```python
from build123d import *

# Parameters (mm, degrees)
F0_W     = 107.6
F0_H     = 53
F1_DEPTH = 14.5
F2_W     = 105.6
F2_H     = 52
F3_DEPTH = 14
F4_SIZE  = 9
F5_W     = 11
F5_H     = 3.2
F6_DEPTH = 1
F7_W     = 15
F7_H     = 6
F8_DEPTH = 1
F9_R     = 2
F10_R    = 4


with BuildPart() as f1:
    # F0 (on Top) → F1 (new body)
    with BuildSketch(Plane.XY):
        Rectangle(F0_W, F0_H)
    extrude(amount=F1_DEPTH)

    # F2 (on face) → F3 (cut)
    with BuildSketch(Plane.XY.offset(14.5)):
        with Locations((0, -0.5)):
            Rectangle(F2_W, F2_H)
    extrude(amount=-F3_DEPTH, mode=Mode.SUBTRACT)

    # F4
    f4_edges = [f1.edges().sort_by_distance(p)[0] for p in [
        (53.8, 0, 0),
        (0, 26.5, 0),
        (-53.8, 0, 0),
        (-52.8, -0.5, 0.5),
        (0, 25.5, 0.5),
        (52.8, -0.5, 0.5),
    ]]
    chamfer(f4_edges, length=F4_SIZE)

    # F5 (on face) → F6 (join)
    with BuildSketch(Plane.XY.offset(14.5)):
        with Locations((-25, 27.1)):
            Rectangle(F5_W, F5_H)
        with Locations((25, 27.1)):
            Rectangle(F5_W, F5_H)
    extrude(amount=F6_DEPTH)

    # F7 (on face) → F8 (join)
    with BuildSketch(Plane.XY.offset(0.5)):
        with Locations((-21.7, -26.5)):
            Rectangle(F7_W, F7_H)
        with Locations((21.7, -26.5)):
            Rectangle(F7_W, F7_H)
    extrude(amount=F8_DEPTH)

    # F9
    f9_edges = [f1.edges().sort_by_distance(p)[0] for p in [
        (-29.2, -29.5, 1),
        (-14.2, -29.5, 1),
        (14.2, -29.5, 1),
        (29.2, -29.5, 1),
        (29.2, -23.5, 1),
        (14.2, -23.5, 1),
        (-29.2, -23.5, 1),
        (-14.2, -23.5, 1),
        (30.5, 28.7, 15),
        (19.5, 28.7, 15),
        (-19.5, 28.7, 15),
        (-30.5, 28.7, 15),
    ]]
    fillet(f9_edges, radius=F9_R)

    # F10
    f10_edges = [f1.edges().sort_by_distance(p)[0] for p in [
        (53.8, 26.5, 11.75),
        (52.8, 25.5, 12),
        (-52.8, 25.5, 12),
        (-53.8, 26.5, 11.75),
    ]]
    fillet(f10_edges, radius=F10_R)


solid = f1.part
```
Geometry check sheet. Reference: the model listing, model coordinates, mm. A direction names the side the tool comes from. Coordinates: 2 decimals unless noted, no trailing zeros. Order: outer loops, then holes, each group sorted by start corner. A loop starts at its lowest first (then second) coordinate and runs counter-clockwise, first axis right, second up. Notation, with made-up numbers: (45, 42) - (99, 42) arc R16 cw to (99, 49) - close; hole circle Ø4 at (70.25, 72). An arc over 180 degrees is marked (long way). Answer in a Markdown table with one row per item. Add a question column.
1. Section check C-C (z = 4.5). Enter the section's corners in (x, y), plus the area to 3 significant figures.
2. Draft check along X on faces 1 (the face through (14.8, -24.07, 1.01)), 2 (the face through (-1, -5, 0.5)), 3 (the face through (52.659, 25.297, 11.211)), 4 (the face through (-53.8, -2, 12)). Enter one of: +X half, -X half, draft (parallel to the pull), parting line (faces both ways), or undercut.
3. Section check D-D (x = 32.5). Enter the section's corners in (y, z).
4. Material ranges on L1, parallel to X at y = 6, z = 10.75; L2, parallel to Y at x = -48.5, z = 12.5; L3, parallel to Z at x = 15, y = -20, recorded low to high. Write a range as [from, to].
5. Gauge pin test, flat ends, axial feed: pin 1 Ø1 at (y, z) = (7.5, 3) entering from +X; pin 2 Ø0.5 at (y, z) = (-26.5, 1) entering from -X; pin 3 Ø0.5 at (y, z) = (-26.5, 1) entering from +X. Record the tip position at first contact, or that the pin passes through.
6. Access from +Z, -Z, +X, -X, +Y, -Y to the whole of each face (thin tool, end or side, straight path). Record for faces 5 (the face through (-48.4, -1.4, 5.1)), 6 (the face through (-14.8, -24.07, 1.01)), 7 (the face through (20.07, 28.1, 15.01)), 8 (the face through (25, 28, 14.5)).
7. Section check A-A (y = -6). Enter the section's corners in (x, z).
8. Section check B-B (x = -17.5). Enter the section's corners in (y, z), plus the area to 3 significant figures.
Data:
| question | item | result |
|---|---|---|
| 1 | outline | (-49.3, -26.5) - (-47.8, -26.5) - (-47.8, 20.5) - (47.8, 20.5) - (47.8, -26.5) - (49.3, -26.5) - (49.3, 22) - (-49.3, 22) - close |
| 1 | area | 289 mm² |
| 2 | face 1 | undercut |
| 2 | face 2 | undercut |
| 2 | face 3 | +X half |
| 2 | face 4 | -X half |
| 3 | outline | (-26.5, 0) - (17.5, 0) - (26.5, 9) - (26.5, 14.5) - (25.5, 14.5) - (25.5, 9.5) - (16.5, 0.5) - (-26.5, 0.5) - close |
| 4 | L1 | x = [-53.8, -52.8], [52.8, 53.8] |
| 4 | L2 | y = [25.5, 26.5] |
| 4 | L3 | z = [0, 0.5] |
| 5 | pin 1 | stops at x = 48.3 |
| 5 | pin 2 | stops at x = -46.05 |
| 5 | pin 3 | stops at x = 46.05 |
| 6 | face 5 | +Z, -Y |
| 6 | face 6 | +Z |
| 6 | face 7 | +Z, -Z, +Y |
| 6 | face 8 | -Z, +X, -X, +Y |
| 7 | outline | (-53.8, 9) - (-44.8, 0) - (44.8, 0) - (53.8, 9) - (53.8, 14.5) - (52.8, 14.5) - (52.8, 9.5) - (43.8, 0.5) - (-43.8, 0.5) - (-52.8, 9.5) - (-52.8, 14.5) - (-53.8, 14.5) - close |
| 8 | outline | (-29.5, 0.5) - (-26.5, 0.5) - (-26.5, 0) - (17.5, 0) - (26.5, 9) - (26.5, 14.5) - (25.5, 14.5) - (25.5, 9.5) - (16.5, 0.5) - (-23.5, 0.5) - (-23.5, 1.5) - (-29.5, 1.5) - close |
| 8 | area | 46.5 mm² |
